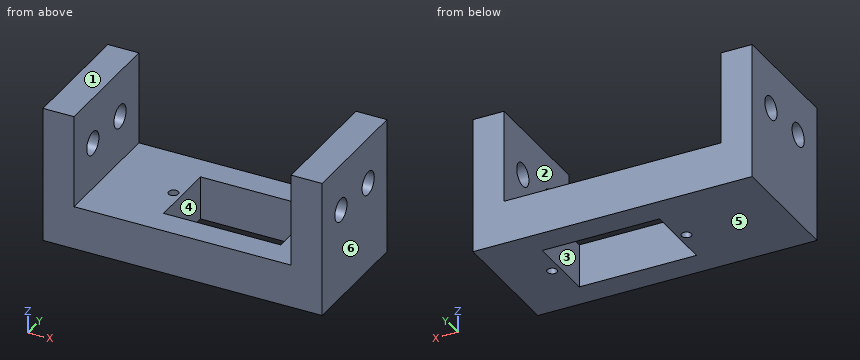
from build123d import *

# Parameters (mm, degrees)
BOSS_EXTRUDE1_DEPTH     = 25.4
CUT_EXTRUDE1_DEPTH      = 60.905780189
CUT_EXTRUDE1_DEPTH_BACK = 60.905780189
SKETCH2_R               = 2.38125
SKETCH3_R               = 1
SKETCH3_W               = 24
SKETCH3_H               = 14.5
CUT_EXTRUDE2_DEPTH      = 48.353291596


with BuildPart() as part:
    # Sketch1 → Boss-Extrude1 (new body)
    with BuildSketch(Plane(origin=(0, 0, 0), x_dir=(1, 0, 0), z_dir=(0, 1, 0))):
        Polygon((-28.575, 8.89), (28.575, 8.89), (28.575, -19.05), (22.225, -19.05), (22.225, 0), (-22.225, 0), (-22.225, -19.05), (-28.575, -19.05), align=None)
    extrude(amount=BOSS_EXTRUDE1_DEPTH)

    # Sketch2 → Cut-Extrude1 (cut, two sides: drawn at the far end of the back side and taken through both)
    with BuildSketch(Plane.ZY.offset(-22.225).offset(-CUT_EXTRUDE1_DEPTH_BACK)):
        with Locations((9.525, 18.034)):
            Circle(SKETCH2_R)
        with Locations(Location((9.525, 7.366, 0), (0, 0, 180))):
            Circle(SKETCH2_R)
    extrude(amount=CUT_EXTRUDE1_DEPTH + CUT_EXTRUDE1_DEPTH_BACK, mode=Mode.SUBTRACT)

    # Sketch3 → Cut-Extrude2 (cut, through all)
    with BuildSketch(Plane(origin=(0, 0, -8.89), x_dir=(-1, 0, 0), z_dir=(0, 0, -1))):
        with Locations((8.5, 12.7)):
            Circle(SKETCH3_R)
        with Locations((-19, 12.7)):
            Circle(SKETCH3_R)
        with Locations((-5.25, 12.7)):
            Rectangle(SKETCH3_W, SKETCH3_H)
    extrude(amount=-CUT_EXTRUDE2_DEPTH, mode=Mode.SUBTRACT)


solid = part.part
The model under review builds one solid part; all positions refer to its coordinate system, in mm. Face numbers are marked on the shaded views. A direction names the side the tool comes from. Round coordinates to 2 decimals unless told otherwise and drop trailing zeros. Loops run counter-clockwise (first coordinate to the right, second up) from the corner with the lowest first, then second, coordinate; pieces in that order, holes last. Notation, with made-up numbers: M -7.5,1.25 L 9.5,1.25 A25 cw 9.5,18.25 Z; hole C -16,83.25 d8. An arc over 180 degrees is marked long. Answer as CSV lines item,"result". Start each with the question number.
Item 1: For the marked faces 1, 2 and 3, list the 3-axis set-ups (+Z, -Z, +X, -X, +Y, -Y) from which the entire face can be reached by the end or side of a thin tool; tool diameter is ignored.
Item 2: Wall thickness on line 1 (X direction, y = 5.75, z = 2.25) (3 decimals); line 2 (Y direction, x = 19, z = -5.75); line 3 (Y direction, x = 12, z = -2.5): over which ranges is each line inside the solid? List them lowest first. Write a range as [from, to].
Item 3: Insertion check: P1, Ø6, axis at y = 16.5, z = 9, coming from the -X side (3 decimals); P2, Ø2.5, axis at x = -8.5, y = 12.7, coming from the +Z side. Each pin has a flat end and moves straight along its axis. Give the tip position at first contact, or say it passes through.
Item 4: Consider section A-A (x = -8.5). Write out the cut boundary in (y, z).
Item 5: Consider section D-D (z = 9). Write out the cut boundary in (x, y) (3 decimals), then the cut area to 3 significant figures.
Item 6: Mouldability with a two-part tool opening along X and no side actions: class the marked faces 4, 5 and 6 as released by +X, released by -X, zero draft, split by the parting line, or undercut.
Item 7: Consider section C-C (y = 12.7). Write out the cut boundary in (x, z) (3 decimals), then the cut area to 3 significant figures.
Item 8: Consider section B-B (z = 14.75). Write out the cut boundary in (x, y) (3 decimals).
Answer:
1,face 1,"+Z, +X, -X, +Y, -Y"
1,face 2,"+Z, +Y, -Y"
1,face 3,"+Z, -Z"
2,line 1,"x = [-28.575, -22.225], [22.225, 28.575]"
2,line 2,"y = [0, 11.7], [13.7, 25.4]"
2,line 3,"y = [0, 5.45], [19.95, 25.4]"
3,P1,"stops at x = -28.575"
3,P2,"stops at z = 0"
4,outline,"M 0,-8.89 L 11.7,-8.89 L 11.7,0 L 0,0 Z; M 13.7,-8.89 L 25.4,-8.89 L 25.4,0 L 13.7,0 Z"
5,outline,"M -28.575,0 L -22.225,0 L -22.225,5.043 L -28.575,5.043 Z; M -28.575,9.689 L -22.225,9.689 L -22.225,15.711 L -28.575,15.711 Z; M -28.575,20.357 L -22.225,20.357 L -22.225,25.4 L -28.575,25.4 Z; M 22.225,0 L 28.575,0 L 28.575,5.043 L 22.225,5.043 Z; M 22.225,9.689 L 28.575,9.689 L 28.575,15.711 L 22.225,15.711 Z; M 22.225,20.357 L 28.575,20.357 L 28.575,25.4 L 22.225,25.4 Z"
5,area,"205 mm^2"
6,face 4,"undercut"
6,face 5,"zero draft"
6,face 6,"released by +X"
7,outline,"M -28.575,-8.89 L -9.5,-8.89 L -9.5,0 L -22.225,0 L -22.225,19.05 L -28.575,19.05 Z; M -7.5,-8.89 L -6.75,-8.89 L -6.75,0 L -7.5,0 Z; M 17.25,-8.89 L 18,-8.89 L 18,0 L 17.25,0 Z; M 20,-8.89 L 28.575,-8.89 L 28.575,19.05 L 22.225,19.05 L 22.225,0 L 20,0 Z"
7,area,"501 mm^2"
8,outline,"M -28.575,0 L -22.225,0 L -22.225,25.4 L -28.575,25.4 Z; M 22.225,0 L 28.575,0 L 28.575,25.4 L 22.225,25.4 Z"
